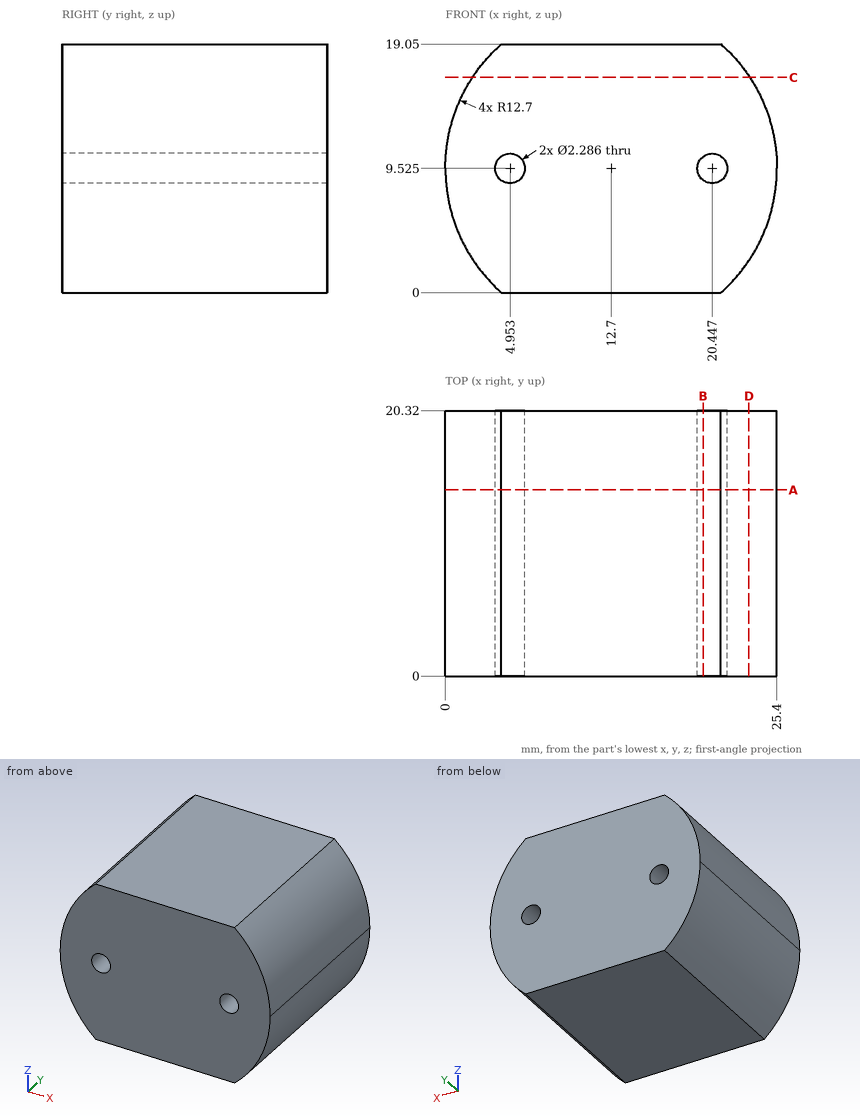
Source: three-view drawing plus pictorial views. Frame: mm from the lowest corner of the part. Give positions to 0.01 mm unless a question says otherwise; leave off trailing zeros. Write each loop counter-clockwise with the first axis right and the second up, starting at its lowest first coordinate (ties: lowest second). Pieces come first, ordered by that corner, then holes. Notation, with made-up numbers: (-28, 13) -> (3, 13) arc R22 ccw to (3, 37) -> close; hole circle Ø6 at (-10, 78). An arc over 180 degrees is marked (long way). Answer in a Markdown table with one row per item.
(1) Section query D-D on x = 23.25. Return loops of the section in (y, z).
Answers below:
| item | result |
|---|---|
| outline | (0, 2.45) -> (20.32, 2.45) -> (20.32, 16.6) -> (0, 16.6) -> close |
(2) Pin query (flat end, axial travel): pin 1 (1 mm diameter, centred on y = 5.5, z = 12, fed in from -X). Return the tip coordinate at first contact, or that it passes through.
Answers below:
| item | result |
|---|---|
| pin 1 | x = 0.15 |
(3) Section query B-B on x = 19.75. Return loops of the section in (y, z), then the cut area to 3 significant figures.
Answers below:
| item | result |
|---|---|
| outline | (0, 0) -> (20.32, 0) -> (20.32, 8.62) -> (0, 8.62) -> close; (0, 10.43) -> (20.32, 10.43) -> (20.32, 19.05) -> (0, 19.05) -> close |
| area | 350 mm^2 |
(4) Section query A-A on y = 14.25. State how many separate pieces and enclosed holes the cut face has, then the cut area to 3 significant figures.
Answers below:
| item | result |
|---|---|
| separate pieces | 1 |
| enclosed holes | 2 |
| area | 425 mm^2 |
(5) Ray query, line 1 along Z through (x, y) = (5, 14); line 2 along X through (y, z) = (4, 10.5); line 3 along X through (y, z) = (14.75, 10). Return the intervals inside material, ascending. Write a range as [from, to].
Answers below:
| item | result |
|---|---|
| line 1 | [0, 8.38], [10.67, 19.05] |
| line 2 | [0.04, 4.36], [5.55, 19.85], [21.04, 25.36] |
| line 3 | [0.01, 3.91], [5.99, 19.41], [21.49, 25.39] |
(6) Section query C-C on z = 16.5. Return loops of the section in (x, y).
Answers below:
| item | result |
|---|---|
| outline | (2.09, 0) -> (23.31, 0) -> (23.31, 20.32) -> (2.09, 20.32) -> close |
